Print and shaded views of the part. All mm, measured from the part's lowest x, y and z. A direction names the side the tool comes from. Give positions to 0.01 mm unless a question says otherwise; leave off trailing zeros. Write each loop counter-clockwise with the first axis right and the second up, starting at its lowest first coordinate (ties: lowest second). Pieces come first, ordered by that corner, then holes. Notation, with made-up numbers: (66, 87) - (106, 87) arc R16 cw to (106, 99) - close; hole circle Ø2 at (-22.5, -39). An arc over 180 degrees is marked (long way). Use one line per item in the form item = value. Start each with the question number.
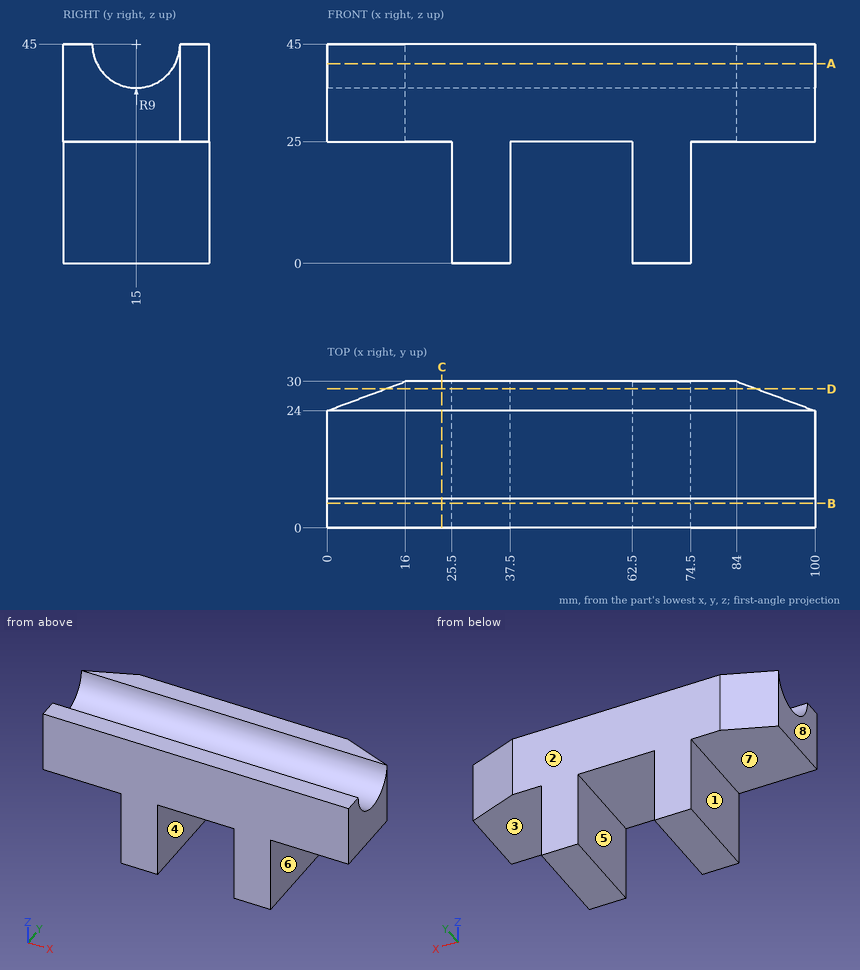
(1) Cut at D-D, the plane y = 28.5. Give the cut face in (x, z), then the cut area to 3 significant figures.
(2) Pin check, flat tips, straight feed: pin 1 Ø1 at (x, y) = (57, 18) entering from -Z; pin 2 Ø1.5 at (x, z) = (89, 34.5) entering from +Y; pin 3 Ø12.5 at (y, z) = (14.5, 16.5) entering from +X; pin 4 Ø5 at (y, z) = (25, 27) entering from +X. Stop position of each tip, or through.
(3) Two-plate mould, pull along X, no slides. Class the marked faces 5, 6, 7 and 8: +X half, -X half, draft (parallel to the pull), parting line (faces both ways), or undercut.
(4) Cut at B-B, the plane y = 5. Give the cut face in (x, z).
(5) Cut at C-C, the plane x = 23.5. Give the cut face in (y, z).
(6) Which spindle directions (+Z, -Z, +X, -X, +Y, -Y) get a long thin tool onto all of the face, cutting with end or side? Do the marked faces 1, 2, 3 and 4. Say none if no direction does.
(7) Wall check: line 1 (X direction, y = 17, z = 20); line 2 (Z direction, x = 90.5, y = 10); line 3 (Z direction, x = 27, y = 14.5). Give the ranges that are in metal, low to high. Write a range as from..to.
(8) Cut at A-A, the plane z = 41. Give the cut face in (x, y), then the cut area to 3 significant figures.
Solution:
q1.outline = (12, 25) - (25.5, 25) - (25.5, 0) - (37.5, 0) - (37.5, 25) - (62.5, 25) - (62.5, 0) - (74.5, 0) - (74.5, 25) - (88, 25) - (88, 45) - (12, 45) - close
q1.area = 2,120 mm2
q2.pin_1 = 25
q2.pin_2 = 28.41
q2.pin_3 = 74.5
q2.pin_4 = 100
q3.face_5 = undercut
q3.face_6 = +X half
q3.face_7 = draft
q3.face_8 = -X half
q4.outline = (0, 25) - (25.5, 25) - (25.5, 0) - (37.5, 0) - (37.5, 25) - (62.5, 25) - (62.5, 0) - (74.5, 0) - (74.5, 25) - (100, 25) - (100, 45) - (0, 45) - close
q5.outline = (0, 25) - (30, 25) - (30, 45) - (24, 45) arc R9 cw to (6, 45) - (0, 45) - close
q6.face_1 = -Z, -X, +Y, -Y
q6.face_2 = +Z, -Z, +X, -X, +Y
q6.face_3 = -Z, +X, +Y, -Y
q6.face_4 = -Z, +Y, -Y
q7.line_1 = 25.5..37.5, 62.5..74.5
q7.line_2 = 25..37.52
q7.line_3 = 0..36.01
q8.outline = (0, 0) - (100, 0) - (100, 6.94) - (0, 6.94) - close; (0, 23.06) - (100, 23.06) - (100, 24) - (84, 30) - (16, 30) - (0, 24) - close
q8.area = 1,290 mm2
